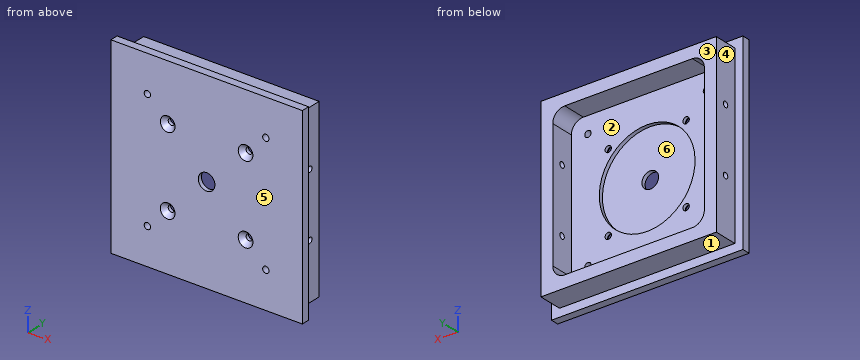
from build123d import *
from OCP.BRepFilletAPI import BRepFilletAPI_MakeChamfer

# Parameters (mm, degrees)
SKETCH1_W                    = 76.2
SKETCH1_H                    = 76.2
BOSS_EXTRUDE1_DEPTH          = 3.175
SKETCH2_W                    = 69.79412
SKETCH2_H                    = 69.79412
SKETCH2_W_2                  = 60.325
SKETCH2_H_2                  = 60.325
BOSS_EXTRUDE2_DEPTH          = 9.525
FILLET1_R                    = 4.7625
SKETCH3_R                    = 19.05
CUT_EXTRUDE1_DEPTH           = 1.5875
SKETCH4_R                    = 3.302
CUT_EXTRUDE2_DEPTH           = 56.015521957
F_39_0_0995_DIAMETER_HOLE1_D = 2.5273
CHAMFER1_SIZE                = 1.905
CHAMFER1_SIZE2               = 1.655991236


with BuildPart() as part:
    # Sketch1 → Boss-Extrude1 (new body)
    with BuildSketch(Plane(origin=(0, 0, 0), x_dir=(1, 0, 0), z_dir=(0, 1, 0))):
        Rectangle(SKETCH1_W, SKETCH1_H)
    extrude(amount=BOSS_EXTRUDE1_DEPTH)

    # Sketch2 → Boss-Extrude2 (add)
    with BuildSketch(Plane(origin=(0, 3.175, 0), x_dir=(1, 0, 0), z_dir=(0, 1, 0))):
        Rectangle(SKETCH2_W, SKETCH2_H)
        Rectangle(SKETCH2_W_2, SKETCH2_H_2, mode=Mode.SUBTRACT)
    extrude(amount=BOSS_EXTRUDE2_DEPTH)

    # Fillet1
    fillet1_edges = [part.edges().sort_by_distance(p)[0] for p in [
        (-30.1625, 7.9375, 30.1625),
        (30.1625, 7.9375, 30.1625),
        (30.1625, 7.9375, -30.1625),
        (-30.1625, 7.9375, -30.1625),
    ]]
    fillet(fillet1_edges, radius=FILLET1_R)

    # Sketch3 → Cut-Extrude1 (cut)
    with BuildSketch(Plane(origin=(0, 3.175, 0), x_dir=(1, 0, 0), z_dir=(0, 1, 0))):
        with Locations(Location((0, 0, 0), (0, 0, 270))):
            Circle(SKETCH3_R)
    extrude(amount=-CUT_EXTRUDE1_DEPTH, mode=Mode.SUBTRACT)

    # Sketch4 → Cut-Extrude2 (cut, through all)
    with BuildSketch(Plane(origin=(0, 1.5875, 0), x_dir=(1, 0, 0), z_dir=(0, 1, 0))):
        with Locations(Location((0, 0, 0), (0, 0, 270))):
            Circle(SKETCH4_R)
    extrude(amount=-CUT_EXTRUDE2_DEPTH, mode=Mode.SUBTRACT)

    # #39 (0.0995) Diameter Hole1 (through all)
    with Locations(Plane(origin=(0, 3.175, 0), x_dir=(1, 0, 0), z_dir=(0, 1, 0))):
        with Locations((15.5, 15.5), (-15.5, 15.5), (-15.5, -15.5), (15.5, -15.5), (-23.57, 23.57), (23.57, 23.57), (23.57, -23.57), (-23.57, -23.57)):
            Hole(F_39_0_0995_DIAMETER_HOLE1_D / 2)

    # Sketch9 → #4-40 Tapped Hole1 (revolve, cut)
    with BuildSketch(Plane(origin=(34.89706, 7.9375, 12.7), x_dir=(0, 0, -1), z_dir=(0, 1, 0))):
        Polygon((0, 0), (0, 7.283152758), (1.1303, 6.604), (1.1303, 0), align=None)
    f_4_40_tapped_hole1 = revolve(axis=Axis((41.24706, 7.9375, 12.7), (-1, 0, 0)), mode=Mode.SUBTRACT)

    # Mirror1: #4-40 Tapped Hole1 across plane
    add(f_4_40_tapped_hole1.mirror(Plane.XY), mode=Mode.SUBTRACT)

    # Mirror2: #4-40 Tapped Hole1 across plane
    add(f_4_40_tapped_hole1.mirror(Plane(origin=(0, 0, 0), x_dir=(0, 0, 1), z_dir=(1, 0, 0))), mode=Mode.SUBTRACT)

    # Mirror2 copy 1 sketch → Mirror2 copy 1 (revolve, cut)
    with BuildSketch(Plane(origin=(-34.89706, 7.9375, -12.7), x_dir=(0, 0, 1), z_dir=(0, 1, 0))):
        Polygon((0, 0), (0, 7.283152758), (1.1303, 6.604), (1.1303, 0), align=None)
    revolve(axis=Axis((-41.24706, 7.9375, -12.7), (1, 0, 0)), mode=Mode.SUBTRACT)

    # Chamfer1: one chamfer whose edges measure the first distance from different faces: ONE call of the kernel's chamfer builder (chamfer() names one face for all edges)
    chamfer1_edges_1 = [part.edges().sort_by_distance(p)[0] for p in [
        (16.76365, 0, 15.5),
    ]]
    chamfer1_side_1 = [part.faces().sort_by_distance(p)[0] for p in [
        (16.76365, 1.5875, 15.5),
    ]]
    chamfer1_edges_2 = [part.edges().sort_by_distance(p)[0] for p in [
        (-14.23635, 0, 15.5),
    ]]
    chamfer1_side_2 = [part.faces().sort_by_distance(p)[0] for p in [
        (-14.23635, 1.5875, 15.5),
    ]]
    chamfer1_edges_3 = [part.edges().sort_by_distance(p)[0] for p in [
        (-14.23635, 0, -15.5),
    ]]
    chamfer1_side_3 = [part.faces().sort_by_distance(p)[0] for p in [
        (-14.23635, 1.5875, -15.5),
    ]]
    chamfer1_edges_4 = [part.edges().sort_by_distance(p)[0] for p in [
        (16.76365, 0, -15.5),
    ]]
    chamfer1_side_4 = [part.faces().sort_by_distance(p)[0] for p in [
        (16.76365, 1.5875, -15.5),
    ]]
    chamfer1 = BRepFilletAPI_MakeChamfer(part.part.solid().wrapped)
    for e in chamfer1_edges_1:
        chamfer1.Add(CHAMFER1_SIZE, CHAMFER1_SIZE2, e.wrapped, chamfer1_side_1[0].wrapped)  # the first distance lies on this face
    for e in chamfer1_edges_2:
        chamfer1.Add(CHAMFER1_SIZE, CHAMFER1_SIZE2, e.wrapped, chamfer1_side_2[0].wrapped)  # the first distance lies on this face
    for e in chamfer1_edges_3:
        chamfer1.Add(CHAMFER1_SIZE, CHAMFER1_SIZE2, e.wrapped, chamfer1_side_3[0].wrapped)  # the first distance lies on this face
    for e in chamfer1_edges_4:
        chamfer1.Add(CHAMFER1_SIZE, CHAMFER1_SIZE2, e.wrapped, chamfer1_side_4[0].wrapped)  # the first distance lies on this face
    add(Compound.cast(chamfer1.Shape()), mode=Mode.REPLACE)


solid = part.part
Source: CAD feature listing. Evaluate the final solid. Frame: model axes, mm. Face numbers are marked on the shaded views. A direction names the side the tool comes from. Give positions to 0.01 mm unless a question says otherwise; leave off trailing zeros. Order: outer loops, then holes, each group sorted by start corner. A loop starts at its lowest first (then second) coordinate and runs counter-clockwise, first axis right, second up. Notation, with made-up numbers: (77, 38) -> (108, 38) arc R26 ccw to (108, 75) -> close; hole circle Ø10 at (-36.5, 77.25). An arc over 180 degrees is marked (long way). Write item = value, one per line.
Q1. Cut plane D-D, the plane z = 15.5. Output: boundary loops of the cut face in (x, y) (1 decimal).
Data:
outline = (-38.1, 0) -> (-18.4, 0) -> (-16.8, 1.9) -> (-16.8, 3.2) -> (-30.2, 3.2) -> (-30.2, 12.7) -> (-34.9, 12.7) -> (-34.9, 3.2) -> (-38.1, 3.2) -> close; (-14.2, 1.9) -> (-12.6, 0) -> (12.6, 0) -> (14.2, 1.9) -> (14.2, 3.2) -> (11.1, 3.2) -> (11.1, 1.6) -> (-11.1, 1.6) -> (-11.1, 3.2) -> (-14.2, 3.2) -> close; (16.8, 1.9) -> (18.4, 0) -> (38.1, 0) -> (38.1, 3.2) -> (34.9, 3.2) -> (34.9, 12.7) -> (30.2, 12.7) -> (30.2, 3.2) -> (16.8, 3.2) -> close
Q2. Cut plane C-C, the plane y = 11.75. Output: boundary loops of the cut face in (x, z) (1 decimal).
Data:
outline = (-34.9, -34.9) -> (34.9, -34.9) -> (34.9, 34.9) -> (-34.9, 34.9) -> close; hole (-30.2, -25.4) arc R4.8 ccw to (-25.4, -30.2) -> (25.4, -30.2) arc R4.8 ccw to (30.2, -25.4) -> (30.2, 25.4) arc R4.8 ccw to (25.4, 30.2) -> (-25.4, 30.2) arc R4.8 ccw to (-30.2, 25.4) -> close
Q3. Pull-direction query (Z, two-part tool) for the marked faces 1, 2 and 3; classes: released by +Z, released by -Z, zero draft, split by the parting line, or undercut.
Data:
face_1 = released by -Z
face_2 = undercut
face_3 = zero draft
Q4. Pin query (flat end, axial travel): pin 1 (5 mm diameter, centred on x = 6, y = 8, fed in from +Z); pin 2 (8 mm diameter, centred on x = 20.5, z = -24.5, fed in from +Y) (3 decimals); pin 3 (2 mm diameter, centred on x = -15.5, z = 15.5, fed in from +Y); pin 4 (3 mm diameter, centred on y = 6.5, z = 14, fed in from +X). Return the tip coordinate at first contact, or that it passes through.
Data:
pin_1 = 34.9
pin_2 = 3.175
pin_3 = through
pin_4 = 34.9
Q5. Material intervals for line 1 (X direction, y = 2.45, z = -23.57); line 2 (X direction, y = 4, z = -0.5), sorted ascending. Write a range as from..to.
Data:
line_1 = -38.1..-24.83, -22.31..22.31, 24.83..38.1
line_2 = -34.9..-30.16, 30.16..34.9
Q6. Cut plane A-A, the plane z = -23.57. Output: boundary loops of the cut face in (x, y) (1 decimal), and give its area (3 significant figures).
Data:
outline = (-38.1, 0) -> (-24.8, 0) -> (-24.8, 3.2) -> (-30.2, 3.2) -> (-30.2, 12.7) -> (-34.9, 12.7) -> (-34.9, 3.2) -> (-38.1, 3.2) -> close; (-22.3, 0) -> (22.3, 0) -> (22.3, 3.2) -> (-22.3, 3.2) -> close; (24.8, 0) -> (38.1, 0) -> (38.1, 3.2) -> (34.9, 3.2) -> (34.9, 12.7) -> (30.2, 12.7) -> (30.2, 3.2) -> (24.8, 3.2) -> close
area = 316 mm^2
Q7. Set-up query: the marked faces 4, 5 and 6. Return all of +Z, -Z, +X, -X, +Y, -Y with unobstructed straight access to the full face (end or side cutting, diameter ignored); none if empty.
Data:
face_4 = +Z, -Z, -X, +Y
face_5 = +Z, -Z, +X, -X, -Y
face_6 = +Y
Q8. Cut plane B-B, the plane x = 20. Output: boundary loops of the cut face in (y, z) (1 decimal), and give its area (3 significant figures).
Data:
outline = (0, -38.1) -> (3.2, -38.1) -> (3.2, -34.9) -> (12.7, -34.9) -> (12.7, -30.2) -> (3.2, -30.2) -> (3.2, 30.2) -> (12.7, 30.2) -> (12.7, 34.9) -> (3.2, 34.9) -> (3.2, 38.1) -> (0, 38.1) -> close
area = 332 mm^2
